Read the model definition and answer for the solid it produces. Units are mm, in the model's axes. Face numbers are marked on the shaded views. A direction names the side the tool comes from. Coordinates: 2 decimals unless noted, no trailing zeros. Order: outer loops, then holes, each group sorted by start corner. A loop starts at its lowest first (then second) coordinate and runs counter-clockwise, first axis right, second up. Notation, with made-up numbers: (85, 5) -> (135, 5) arc R16 cw to (135, 31) -> close; hole circle Ø4 at (52, 58). An arc over 180 degrees is marked (long way). Answer as a JSON object with one key per item and string values. Group by question number.
1) Consider L1, parallel to Y at x = 25, z = -23 (3 decimals); L2, parallel to Y at x = -7, z = -7 (3 decimals); L3, parallel to Z at x = -1.5, y = -14. Determine where each line is inside the solid, lowest interval first.
2) A tool of negligible diameter and unlimited length cuts with its end or side. For the marked faces 1, 2 and 3, from which of +Z, -Z, +X, -X, +Y, -Y can it reach the whole face along a straight path? Write none if from no direction.
3) Section B-B on x = 15 is taken. Determine the outline of the cut face in (y, z) (3 decimals).
4) Determine the mould class of the marked faces 4, 5 and 6 for opening direction X: released by +X, released by -X, zero draft, split by the parting line, or undercut.
5) Section D-D on y = 7 is taken. Determine the outline of the cut face in (x, z).
6) Section A-A on x = 5 is taken. Determine the outline of the cut face in (y, z) (3 decimals).
7) Section C-C on z = 4 is taken. Determine the outline of the cut face in (x, y) (3 decimals).
8) Given pin 1 (5 mm diameter, centred on x = 0.5, z = -6.5, fed in from -Y) (3 decimals); pin 2 (2 mm diameter, centred on y = -19, z = -19, fed in from +X); pin 3 (6.5 mm diameter, centred on x = 25, y = -17.87, fed in from +Z); pin 4 (1.6 mm diameter, centred on x = 15.5, y = -10, fed in from +Z), each flat-ended and moving along its own axis, determine where each tip first touches the part or whether it passes through.
from build123d import *

# Parameters (mm, degrees)
BOSS_EXTRUDE1_DEPTH = 30
SKETCH2_R           = 4.125
CUT_EXTRUDE1_DEPTH  = 53.821779702
SKETCH3_W           = 36
SKETCH3_H           = 3.997849999
BOSS_EXTRUDE2_DEPTH = 10
SKETCH4_W           = 36
SKETCH4_H           = 4
BOSS_EXTRUDE3_DEPTH = 10
SKETCH5_R           = 5
BOSS_EXTRUDE4_DEPTH = 12.6
BOSS_EXTRUDE5_START = 7
SKETCH6_W           = 30
SKETCH6_H           = 22.5
SKETCH6_R           = 4.125
BOSS_EXTRUDE5_DEPTH = 7
SKETCH8_R           = 5
SKETCH8_R_2         = 3.5
CUT_EXTRUDE2_DEPTH  = 10.1
SKETCH9_W           = 7
SKETCH9_H           = 22.5
BOSS_EXTRUDE6_DEPTH = 10
SKETCH10_W          = 7
SKETCH10_H          = 22.5
BOSS_EXTRUDE7_DEPTH = 10


with BuildPart() as part:
    # Sketch1 → Boss-Extrude1 (new body)
    with BuildSketch(Plane(origin=(0, 0, 0), x_dir=(0, 0, -1), z_dir=(1, 0, 0))):
        Polygon((16.698859865, -1.874995608), (-15.301140135, -1.874995608), (-15.301140135, -5.874995608), (-6.301140135, -5.874995608), (-5.301140135, -6.674995608), (6.198859865, -6.674995608), (7.198859865, -5.874995608), (16.198859865, -5.874995608), (17.698859865, -6.874995608), (17.698859865, -12.374995608), (16.698859865, -13.374995608), (16.698859865, -24.374995608), (20.698859865, -24.374995608), (20.698859865, -1.874995608), align=None)
    extrude(amount=BOSS_EXTRUDE1_DEPTH)

    # Sketch2 → Cut-Extrude1 (cut, through all)
    with BuildSketch(Plane(origin=(0, 0, -20.698859865), x_dir=(-1, 0, 0), z_dir=(0, 0, -1))):
        with Locations((-25, -17.874995608)):
            Circle(SKETCH2_R)
        with Locations(Location((-5, -17.874995608, 0), (0, 0, 90))):
            Circle(SKETCH2_R)
    extrude(amount=-CUT_EXTRUDE1_DEPTH, mode=Mode.SUBTRACT)

    # Sketch3 → Boss-Extrude2 (add)
    with BuildSketch(Plane.ZY):
        with Locations((-2.698859865, -3.873920608)):
            Rectangle(SKETCH3_W, SKETCH3_H)
    extrude(amount=BOSS_EXTRUDE2_DEPTH)

    # Sketch4 → Boss-Extrude3 (add)
    with BuildSketch(Plane(origin=(30, 0, 0), x_dir=(0, 0, -1), z_dir=(1, 0, 0))):
        with Locations((2.698859865, -3.874995608)):
            Rectangle(SKETCH4_W, SKETCH4_H)
    extrude(amount=BOSS_EXTRUDE3_DEPTH)

    # Sketch5 → Boss-Extrude4 (add)
    with BuildSketch(Plane(origin=(0, -1.874995608, 0), x_dir=(1, 0, 0), z_dir=(0, 1, 0))):
        with Locations((35, 11.198859865)):
            Circle(SKETCH5_R)
        with Locations(Location((-5, 11.198859865, 0), (0, 0, 90))):
            Circle(SKETCH5_R)
    extrude(amount=BOSS_EXTRUDE4_DEPTH)

    # Sketch6 → Boss-Extrude5 (add)
    with BuildSketch(Plane(origin=(0, 0, -20.698859865), x_dir=(-1, 0, 0), z_dir=(0, 0, -1)).offset(BOSS_EXTRUDE5_START)):
        with Locations((-15, -13.124995608)):
            Rectangle(SKETCH6_W, SKETCH6_H)
        with Locations(Location((-25, -17.874995608, 0), (0, 0, 90))):
            Circle(SKETCH6_R, mode=Mode.SUBTRACT)
        with Locations(Location((-5, -17.874995608, 0), (0, 0, 90))):
            Circle(SKETCH6_R, mode=Mode.SUBTRACT)
    extrude(amount=-BOSS_EXTRUDE5_DEPTH)

    # Sketch8 → Cut-Extrude2 (cut)
    # profile 1 of 2: a face of its own
    with BuildSketch(Plane(origin=(0, -0.874995608, 0), x_dir=(1, 0, 0), z_dir=(0, 1, 0))):
        with Locations(Location((-5, 11.198859865, 0), (0, 0, 180))):
            Circle(SKETCH8_R)
        with Locations(Location((-5, 11.198859865, 0), (0, 0, 90))):
            Circle(SKETCH8_R_2, mode=Mode.SUBTRACT)
    # profile 2 of 2: a face of its own
    with BuildSketch(Plane(origin=(0, -0.874995608, 0), x_dir=(1, 0, 0), z_dir=(0, 1, 0))):
        with Locations((35, 11.198859865)):
            Circle(SKETCH8_R)
        with Locations(Location((35, 11.198859865, 0), (0, 0, 90))):
            Circle(SKETCH8_R_2, mode=Mode.SUBTRACT)
    extrude(amount=CUT_EXTRUDE2_DEPTH, mode=Mode.SUBTRACT)

    # Sketch9 → Boss-Extrude6 (add)
    with BuildSketch(Plane(origin=(30, 0, 0), x_dir=(0, 0, -1), z_dir=(1, 0, 0))):
        with Locations((24.198859865, -13.124995608)):
            Rectangle(SKETCH9_W, SKETCH9_H)
    extrude(amount=BOSS_EXTRUDE6_DEPTH)

    # Sketch10 → Boss-Extrude7 (add)
    with BuildSketch(Plane.ZY):
        with Locations((-24.198859865, -13.124995608)):
            Rectangle(SKETCH10_W, SKETCH10_H)
    extrude(amount=BOSS_EXTRUDE7_DEPTH)


solid = part.part
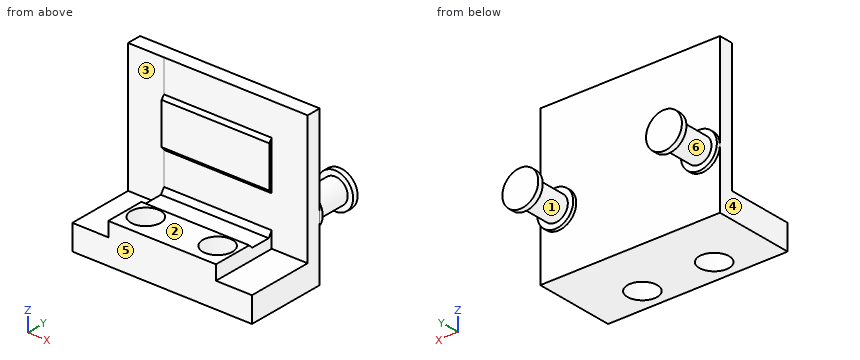
Worked answers:
{
 "1": {"L1": "y = -24.375 to -22, -13.75 to -1.875", "L2": "y = -5.873 to -0.875, 9.225 to 10.725", "L3": "z = -27.7 to -20.7"},
 "2": {"face 1": "none", "face 2": "+Z, +X, -X, -Y", "face 3": "+Z, -X, -Y"},
 "3": {"outline": "(-24.375, -27.699) -> (-1.875, -27.699) -> (-1.875, 15.301) -> (-5.875, 15.301) -> (-5.875, 6.301) -> (-6.675, 5.301) -> (-6.675, -6.199) -> (-5.875, -7.199) -> (-5.875, -16.199) -> (-6.875, -17.699) -> (-12.375, -17.699) -> (-13.375, -16.699) -> (-24.375, -16.699) -> close"},
 "4": {"face 4": "released by -X", "face 5": "zero draft", "face 6": "undercut"},
 "5": {"outline": "circle Ø7 at (-5, -11.2); circle Ø7 at (35, -11.2)"},
 "6": {"outline": "(-24.375, -27.699) -> (-22, -27.699) -> (-22, -16.699) -> (-24.375, -16.699) -> close; (-13.75, -27.699) -> (-1.875, -27.699) -> (-1.875, 15.301) -> (-5.875, 15.301) -> (-5.875, 6.301) -> (-6.675, 5.301) -> (-6.675, -6.199) -> (-5.875, -7.199) -> (-5.875, -16.199) -> (-6.875, -17.699) -> (-12.375, -17.699) -> (-13.375, -16.699) -> (-13.75, -16.699) -> close"},
 "7": {"outline": "(-10, -5.873) -> (0, -5.873) -> (0, -6.675) -> (30, -6.675) -> (30, -5.875) -> (40, -5.875) -> (40, -1.875) -> (-10, -1.875) -> close"},
 "8": {"pin 1": "stops at y = -6.675", "pin 2": "stops at x = 30", "pin 3": "passes through", "pin 4": "stops at z = -17.7"}
}
